Verification items for the finished model (mm, model axes). Face numbers are marked on the shaded views. A direction names the side the tool comes from. Give positions to 0.01 mm unless a question says otherwise; leave off trailing zeros. Write each loop counter-clockwise with the first axis right and the second up, starting at its lowest first coordinate (ties: lowest second). Pieces come first, ordered by that corner, then holes. Notation, with made-up numbers: (61.5, -33) - (110.5, -33) arc R22 ccw to (110.5, -18) - close; hole circle Ø10 at (-22, 11.5). An arc over 180 degrees is marked (long way). Put each result on its own line as item: value.
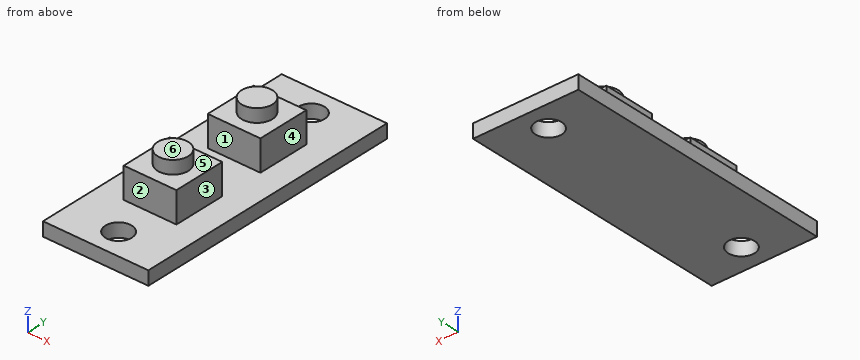
from build123d import *

# Parameters (mm, degrees)
SKETCH1_W               = 12.192
SKETCH1_H               = 31.75
BOSS_EXTRUDE1_DEPTH     = 1.6002
SKETCH2_W               = 6.096
SKETCH2_H               = 6.096
BOSS_EXTRUDE2_DEPTH     = 3.556
SKETCH3_R               = 1.778
BOSS_EXTRUDE3_DEPTH     = 1.524
CUT_EXTRUDE1_DEPTH      = 18.747767212
CUT_EXTRUDE1_DEPTH_BACK = 18.747767212
SKETCH4_R               = 1.524


with BuildPart() as part:
    # Sketch1 → Boss-Extrude1 (new body)
    with BuildSketch(Plane.XY):
        Rectangle(SKETCH1_W, SKETCH1_H)
    extrude(amount=BOSS_EXTRUDE1_DEPTH)

    # Sketch2 → Boss-Extrude2 (add)
    with BuildSketch(Plane.XY.offset(1.6002)):
        with Locations((0, 5.588)):
            Rectangle(SKETCH2_W, SKETCH2_H)
        with Locations((0, -5.588)):
            Rectangle(SKETCH2_W, SKETCH2_H)
    extrude(amount=BOSS_EXTRUDE2_DEPTH)

    # Sketch3 → Boss-Extrude3 (add)
    with BuildSketch(Plane.XY.offset(5.1562)):
        with Locations(Location((0, 5.588, 0), (0, 0, 180))):
            Circle(SKETCH3_R)
        with Locations(Location((0, -5.588, 0), (0, 0, 180))):
            Circle(SKETCH3_R)
    extrude(amount=BOSS_EXTRUDE3_DEPTH)

    # Sketch4 → Cut-Extrude1 (cut, two sides: drawn at the far end of the back side and taken through both)
    with BuildSketch(Plane.XY.offset(1.6002).offset(-CUT_EXTRUDE1_DEPTH_BACK)):
        with Locations((0, 12.827)):
            Circle(SKETCH4_R)
        with Locations((0, -12.827)):
            Circle(SKETCH4_R)
    extrude(amount=CUT_EXTRUDE1_DEPTH + CUT_EXTRUDE1_DEPTH_BACK, mode=Mode.SUBTRACT)


solid = part.part
Q1. Section check D-D, the plane y = 12.5. Record the cut outline in (x, z), plus the area to 3 significant figures.
Answers follow:
outline: (-6.1, 0) - (-1.49, 0) - (-1.49, 1.6) - (-6.1, 1.6) - close; (1.49, 0) - (6.1, 0) - (6.1, 1.6) - (1.49, 1.6) - close
area: 14.7 mm2
Q2. Scan lines: line 1 along Y through (x, z) = (0, 1.3) (3 decimals); line 2 along Y through (x, z) = (2.5, 3.75); line 3 along X through (y, z) = (6.5, 5.75). Record each from-to range of solid material in increasing order.
Answers follow:
line 1: y = -15.875 to -14.351, -11.303 to 11.303, 14.351 to 15.875
line 2: y = -8.64 to -2.54, 2.54 to 8.64
line 3: x = -1.53 to 1.53
Q3. Go/stop test with flat-tipped pins: pin 1 Ø1 at (x, z) = (-1.5, 3.5) entering from +Y; pin 2 Ø1.5 at (x, y) = (-4, -4.5) entering from -Z; pin 3 Ø3.5 at (x, y) = (0, -12.827) entering from +Z; pin 4 Ø3 at (y, z) = (6, 4) entering from -X. Record where each tip stops, or that it passes through.
Answers follow:
pin 1: stops at y = 8.64
pin 2: stops at z = 0
pin 3: stops at z = 1.6
pin 4: stops at x = -3.05
Q4. Section check C-C, the plane x = -2.25. Record the cut outline in (y, z) (3 decimals).
Answers follow:
outline: (-15.875, 0) - (15.875, 0) - (15.875, 1.6) - (8.636, 1.6) - (8.636, 5.156) - (2.54, 5.156) - (2.54, 1.6) - (-2.54, 1.6) - (-2.54, 5.156) - (-8.636, 5.156) - (-8.636, 1.6) - (-15.875, 1.6) - close
Q5. Section check B-B, the plane x = 0. Record the cut outline in (y, z) (3 decimals), plus the area to 3 significant figures.
Answers follow:
outline: (-15.875, 0) - (-14.351, 0) - (-14.351, 1.6) - (-15.875, 1.6) - close; (-11.303, 0) - (11.303, 0) - (11.303, 1.6) - (8.636, 1.6) - (8.636, 5.156) - (7.366, 5.156) - (7.366, 6.68) - (3.81, 6.68) - (3.81, 5.156) - (2.54, 5.156) - (2.54, 1.6) - (-2.54, 1.6) - (-2.54, 5.156) - (-3.81, 5.156) - (-3.81, 6.68) - (-7.366, 6.68) - (-7.366, 5.156) - (-8.636, 5.156) - (-8.636, 1.6) - (-11.303, 1.6) - close; (14.351, 0) - (15.875, 0) - (15.875, 1.6) - (14.351, 1.6) - close
area: 95.2 mm2
Q6. Section check A-A, the plane z = 3.5. Record the cut outline in (x, y).
Answers follow:
outline: (-3.05, -8.64) - (3.05, -8.64) - (3.05, -2.54) - (-3.05, -2.54) - close; (-3.05, 2.54) - (3.05, 2.54) - (3.05, 8.64) - (-3.05, 8.64) - close
Q7. Release check for a two-part mould opening along Y. For the marked faces 1, 2 and 3 record: released by +Y, released by -Y, zero draft, split by the parting line, or undercut.
Answers follow:
face 1: undercut
face 2: released by -Y
face 3: zero draft
Q8. Set-up check for the marked faces 4, 5 and 6: record each of +Z, -Z, +X, -X, +Y, -Y from which the full face is reachable in a straight line by a thin tool's end or side.
Answers follow:
face 4: +Z, +X, +Y, -Y
face 5: +Z
face 6: +Z, +X, -X, +Y, -Y
